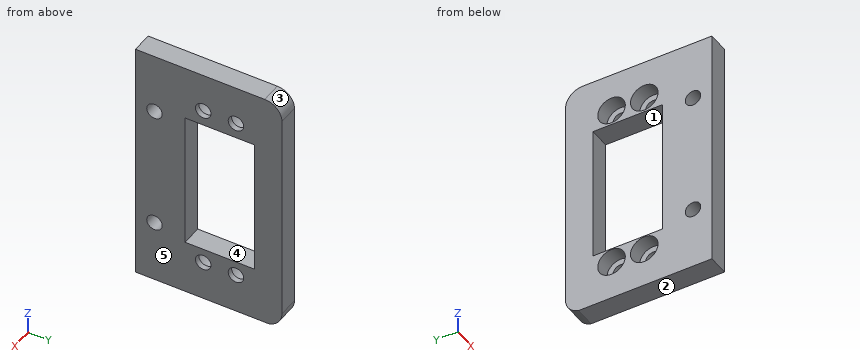
from build123d import *

# Parameters (mm, degrees)
SKETCH1_W                                           = 40.2
SKETCH1_H                                           = 20.1
BOSS_EXTRUDE1_DEPTH                                 = 6
CBORE_FOR_M4_HEX_SOCKET_HEAD_CAP_SCREW1_D           = 4.5
CBORE_FOR_M4_HEX_SOCKET_HEAD_CAP_SCREW1_CBORE_D     = 8
CBORE_FOR_M4_HEX_SOCKET_HEAD_CAP_SCREW1_CBORE_DEPTH = 4.4
M4_CLEARANCE_HOLE1_D                                = 4.5


with BuildPart() as part:
    # Sketch1 → Boss-Extrude1 (new body)
    with BuildSketch(Plane(origin=(0, 0, 0), x_dir=(0, 0, -1), z_dir=(1, 0, 0))):
        with BuildLine():
            Line((-36.096117968, -19.95), (-36.096117968, 17.55))
            ThreePointArc((-36.096117968, 17.55), (-34.631651874, 21.085533906), (-31.096117968, 22.55))
            Line((-31.096117968, 22.55), (31.096117968, 22.55))
            ThreePointArc((31.096117968, 22.55), (34.173179015, 21.49102719), (35.946830469, 18.762678125))
            Line((35.946830469, 18.762678125), (35.946830469, -19.95))
            Line((35.946830469, -19.95), (-36.096117968, -19.95))
        make_face()
        with Locations((0, 4.5)):
            Rectangle(SKETCH1_W, SKETCH1_H, mode=Mode.SUBTRACT)
    extrude(amount=BOSS_EXTRUDE1_DEPTH)

    # CBORE for M4 Hex Socket Head Cap Screw1 (through all)
    with Locations(Plane(origin=(0, -170.712474926, -177.829982134), x_dir=(0, 0, 1), z_dir=(-1, 0, 0))):
        with Locations((202.479982134, 170.412474926), (202.479982134, 179.912474926), (153.479982134, 170.412474926), (153.479982134, 179.912474926)):
            CounterBoreHole(CBORE_FOR_M4_HEX_SOCKET_HEAD_CAP_SCREW1_D / 2, CBORE_FOR_M4_HEX_SOCKET_HEAD_CAP_SCREW1_CBORE_D / 2, CBORE_FOR_M4_HEX_SOCKET_HEAD_CAP_SCREW1_CBORE_DEPTH)

    # M4 Clearance Hole1 (through all)
    with Locations(Plane(origin=(0, -170.712474926, -177.829982134), x_dir=(0, 0, 1), z_dir=(-1, 0, 0))):
        with Locations((160.229982134, 156.262474926), (196.229982134, 156.262474926)):
            Hole(M4_CLEARANCE_HOLE1_D / 2)


solid = part.part
Read the model definition and answer for the solid it produces. Units are mm, in the model's axes. Face numbers are marked on the shaded views. A direction names the side the tool comes from. Give positions to 0.01 mm unless a question says otherwise; leave off trailing zeros. Write each loop counter-clockwise with the first axis right and the second up, starting at its lowest first coordinate (ties: lowest second). Pieces come first, ordered by that corner, then holes. Notation, with made-up numbers: M -33.75,27 L -25.75,27 A19 ccw -25.75,62 Z; hole C 53.25,-5 d1. An arc over 180 degrees is marked long. One line per item, written item: value. Start each with the question number.
(1) Determine the mould class of the marked faces 1, 2 and 3 for opening direction Z: pulls with the +Z half, pulls with the -Z half, needs draft (parallel to the pull), parting line crosses it, or undercut.
(2) Find section D-D (y = 9.2). Determine the outline of the cut face in (x, z), plus the area to 3 significant figures.
(3) A tool of negligible diameter and unlimited length cuts with its end or side. For the marked faces 4 and 5, from which of +Z, -Z, +X, -X, +Y, -Y can it reach the whole face along a straight path? Write none if from no direction.
(4) Find section C-C (x = 3.45). Determine the outline of the cut face in (y, z).
(5) A flat-ended cylindrical pin translates along its axis: pin 1 Ø2.5 at (y, z) = (10, 24) entering from -X. Find the tip coordinate at first contact, or state that the pin passes through.
(6) Find the intervals of material crossed by line 1 (Y direction, x = 5.6, z = -24.35); line 2 (Z direction, x = 5.4, y = 9.2); line 3 (Y direction, x = 1.85, z = 1), in increasing order.
(7) Find section B-B (y = -14.45). Determine the outline of the cut face in (x, z).
(8) Find section A-A (z = 24.65). Determine the outline of the cut face in (x, y), plus the area to 3 significant figures.
Results below:
1. face 1: undercut
1. face 2: pulls with the -Z half
1. face 3: pulls with the +Z half
2. outline: M 0,-35.95 L 6,-35.95 L 6,-26.6 L 4.4,-26.6 L 4.4,-28.35 L 0,-28.35 Z; M 0,-20.35 L 4.4,-20.35 L 4.4,-22.1 L 6,-22.1 L 6,-20.1 L 0,-20.1 Z; M 0,20.1 L 6,20.1 L 6,22.4 L 4.4,22.4 L 4.4,20.65 L 0,20.65 Z; M 0,28.65 L 4.4,28.65 L 4.4,26.9 L 6,26.9 L 6,36.1 L 0,36.1 Z
2. area: 106 mm^2
3. face 4: +X, -X
3. face 5: +Z, -Z, +X, +Y, -Y
4. outline: M -19.95,-35.95 L 18.76,-35.95 A5 ccw 22.55,-31.1 L 22.55,31.1 A5 ccw 17.55,36.1 L -19.95,36.1 Z; hole C -14.45,-17.6 d4.5; hole C -14.45,18.4 d4.5; hole M -5.55,-20.1 L 14.55,-20.1 L 14.55,20.1 L -5.55,20.1 Z; hole C -0.3,-24.35 d8; hole C -0.3,24.65 d8; hole C 9.2,-24.35 d8; hole C 9.2,24.65 d8
5. pin 1: stops at x = 4.4
6. line 1: y = -19.95 to -2.55, 1.95 to 6.95, 11.45 to 22.55
6. line 2: z = -35.95 to -26.6, -22.1 to -20.1, 20.1 to 22.4, 26.9 to 36.1
6. line 3: y = -19.95 to -5.55, 14.55 to 22.55
7. outline: M 0,-35.95 L 6,-35.95 L 6,-19.85 L 0,-19.85 Z; M 0,-15.35 L 6,-15.35 L 6,16.15 L 0,16.15 Z; M 0,20.65 L 6,20.65 L 6,36.1 L 0,36.1 Z
8. outline: M 0,-19.95 L 6,-19.95 L 6,-2.55 L 4.4,-2.55 L 4.4,-4.3 L 0,-4.3 Z; M 0,3.7 L 4.4,3.7 L 4.4,1.95 L 6,1.95 L 6,6.95 L 4.4,6.95 L 4.4,5.2 L 0,5.2 Z; M 0,13.2 L 4.4,13.2 L 4.4,11.45 L 6,11.45 L 6,22.55 L 0,22.55 Z
8. area: 170 mm^2
